Build history of the part. All positions in model axes, mm. Face numbers are marked on the shaded views. A direction names the side the tool comes from. Round coordinates to 2 decimals unless told otherwise and drop trailing zeros. Order: outer loops, then holes, each group sorted by start corner. A loop starts at its lowest first (then second) coordinate and runs counter-clockwise, first axis right, second up. Notation, with made-up numbers: (-29, 50.5) -> (23, 50.5) arc R16 cw to (23, 67.5) -> close; hole circle Ø4 at (75, 77). An arc over 180 degrees is marked (long way). Answer as a JSON object with one key per item and string values.
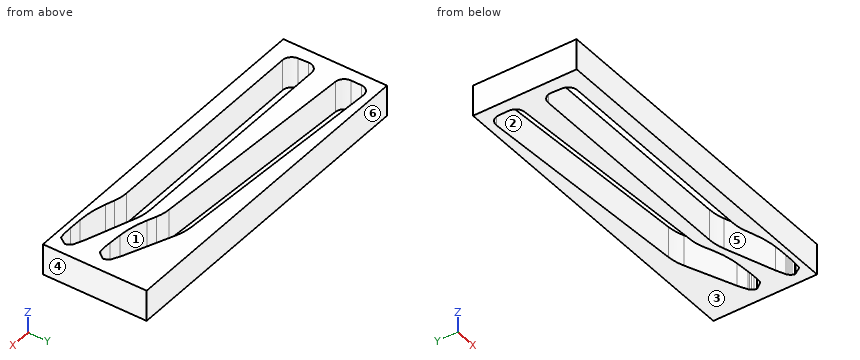
from build123d import *

# Parameters (mm, degrees)
SKETCH1_W           = 32
SKETCH1_H           = 10
BOSS_EXTRUDE1_DEPTH = 3


with BuildPart() as part:
    # Sketch1 → Boss-Extrude1 (new body)
    with BuildSketch(Plane.XY):
        Rectangle(SKETCH1_W, SKETCH1_H)
        with BuildLine():
            Line((7.508183749, -0.761607487), (-13.867203265, -0.724177951))
            ThreePointArc((-13.867203265, -0.724177951), (-14.512395102, -0.999943521), (-14.756643634, -1.657713853))
            Line((-14.756643634, -1.657713853), (-14.706591665, -2.655537266))
            ThreePointArc((-14.706591665, -2.655537266), (-14.431377295, -3.255171805), (-13.818707983, -3.5))
            Line((-13.818707983, -3.5), (6.937095785, -3.5))
            ThreePointArc((6.937095785, -3.5), (7.597596174, -3.554033013), (8.240533164, -3.714695258))
            Line((8.240533164, -3.714695258), (9.052328165, -3.989582288))
            ThreePointArc((9.052328165, -3.989582288), (10.41628769, -4.333930654), (11.817489406, -4.458811135))
            Line((11.817489406, -4.458811135), (13.078294798, -4.471023796))
            ThreePointArc((13.078294798, -4.471023796), (13.681851068, -4.457737599), (14.283353389, -4.406243399))
            Line((14.283353389, -4.406243399), (14.372039696, -4.395810789))
            ThreePointArc((14.372039696, -4.395810789), (14.475481789, -4.359873847), (14.554181178, -4.28372835))
            Line((14.554181178, -4.28372835), (14.962805958, -3.66627609))
            ThreePointArc((14.962805958, -3.66627609), (14.970850873, -3.64453799), (14.968401274, -3.621488801))
            Line((14.968401274, -3.621488801), (14.889319766, -3.39508526))
            ThreePointArc((14.889319766, -3.39508526), (14.851890355, -3.317474793), (14.797978781, -3.25025956))
            Line((14.797978781, -3.25025956), (14.680939758, -3.134135777))
            ThreePointArc((14.680939758, -3.134135777), (14.626648009, -3.089415012), (14.565060551, -3.055436699))
            Line((14.565060551, -3.055436699), (13.68837555, -2.672614052))
            Line((13.68837555, -2.672614052), (9.097693662, -1.037644589))
            ThreePointArc((9.097693662, -1.037644589), (8.314712232, -0.83183031), (7.508183749, -0.761607487))
        make_face(mode=Mode.SUBTRACT)
        with BuildLine():
            Line((7.413496434, 3.116023179), (-13.933174328, 4.224273311))
            ThreePointArc((-13.933174328, 4.224273311), (-14.591371345, 3.981176945), (-14.868266258, 3.336468978))
            Line((-14.868266258, 3.336468978), (-14.868266258, 2.337391022))
            ThreePointArc((-14.868266258, 2.337391022), (-14.623438064, 1.724721711), (-14.023803524, 1.449507341))
            Line((-14.023803524, 1.449507341), (6.705937155, 0.409679726))
            ThreePointArc((6.705937155, 0.409679726), (7.362901198, 0.322624707), (7.996981968, 0.129954245))
            Line((7.996981968, 0.129954245), (8.793986262, -0.185257046))
            ThreePointArc((8.793986262, -0.185257046), (10.138981841, -0.597504878), (11.532167784, -0.792426178))
            Line((11.532167784, -0.792426178), (12.790778149, -0.867787535))
            ThreePointArc((12.790778149, -0.867787535), (13.394242147, -0.884755081), (13.997568925, -0.863459703))
            Line((13.997568925, -0.863459703), (14.086666523, -0.857483214))
            ThreePointArc((14.086666523, -0.857483214), (14.191779099, -0.826773657), (14.274194414, -0.754666471))
            Line((14.274194414, -0.754666471), (14.713239307, -0.158460897))
            ThreePointArc((14.713239307, -0.158460897), (14.722363159, -0.137153129), (14.721071357, -0.114010163))
            Line((14.721071357, -0.114010163), (14.653431554, 0.116070922))
            ThreePointArc((14.653431554, 0.116070922), (14.619937284, 0.195459078), (14.569460767, 0.265290779))
            Line((14.569460767, 0.265290779), (14.458386298, 0.387132185))
            ThreePointArc((14.458386298, 0.387132185), (14.406403152, 0.434516711), (14.34659528, 0.471537776))
            Line((14.34659528, 0.471537776), (13.490189844, 0.897800019))
            Line((13.490189844, 0.897800019), (8.987181446, 2.760701173))
            ThreePointArc((8.987181446, 2.760701173), (8.215494123, 3.00548294), (7.413496434, 3.116023179))
        make_face(mode=Mode.SUBTRACT)
    extrude(amount=BOSS_EXTRUDE1_DEPTH)


solid = part.part
1) Cut at A-A, the plane x = 6. Give the cut face in (y, z).
Checked values:
{"outline": "(-5, 0) -> (-3.5, 0) -> (-3.5, 3) -> (-5, 3) -> close; (-0.76, 0) -> (0.45, 0) -> (0.45, 3) -> (-0.76, 3) -> close; (3.19, 0) -> (5, 0) -> (5, 3) -> (3.19, 3) -> close"}
2) Cut at C-C, the plane z = 0.55. Count the separate pieces of the cut face and the enclosed holes in it, plus the area to 3 significant figures.
Checked values:
{"separate pieces": "1", "enclosed holes": "2", "area": "162 mm²"}
3) Cut at D-D, the plane x = 2.5. Give the cut face in (y, z).
Checked values:
{"outline": "(-5, 0) -> (-3.5, 0) -> (-3.5, 3) -> (-5, 3) -> close; (-0.75, 0) -> (0.62, 0) -> (0.62, 3) -> (-0.75, 3) -> close; (3.37, 0) -> (5, 0) -> (5, 3) -> (3.37, 3) -> close"}
4) Pull direction X, two halves, no side cores. Call the marked faces 1, 2, 3 and 4: pulls with the +X half, pulls with the -X half, needs draft (parallel to the pull), parting line crosses it, or undercut.
Checked values:
{"face 1": "undercut", "face 2": "undercut", "face 3": "needs draft", "face 4": "pulls with the +X half"}
5) Cut at B-B, the plane y = 1.75. Give the cut face in (x, z).
Checked values:
{"outline": "(-16, 0) -> (-14.65, 0) -> (-14.65, 3) -> (-16, 3) -> close; (11.43, 0) -> (16, 0) -> (16, 3) -> (11.43, 3) -> close"}
6) Probe L1, parallel to Y at x = 11, z = 0.2; L2, parallel to Y at x = -8, z = 1.95; L3, parallel to X at y = 2, z = 2.8. List the from-to ranges inside material, lowest first. Write a range as from..to.
Checked values:
{"L1": "y = -5..-4.41, -1.72..-0.74, 1.93..5", "L2": "y = -5..-3.5, -0.73..1.15, 3.92..5", "L3": "x = -16..-14.8, 10.83..16"}
7) Which spindle directions (+Z, -Z, +X, -X, +Y, -Y) get a long thin tool onto all of the face, cutting with end or side? Do the marked faces 5 and 6. Say none if no direction does.
Checked values:
{"face 5": "+Z, -Z", "face 6": "+Z, -Z, +X, -X, +Y"}
